```python
from build123d import *

# Parameters (mm, degrees)
F0_R     = 2
F1_DEPTH = 4
F3_DEPTH = 25
F4_R     = 0.99999
F5_DEPTH = 23
F7_START = 24
F6_W     = 30
F6_H     = 37
F7_DEPTH = 6
F9_DEPTH = 25


# Not quite as in the source:
# - a fillet or chamfer is up to 0.001 mm smaller than in the source, because OpenCascade refuses the exact size


with BuildPart() as f1:
    # F0 (on Top) → F1 (new body)
    with BuildSketch(Plane.XY):
        with BuildLine():
            Line((28.5, 21), (-28.5, 21))
            ThreePointArc((-28.5, 21), (-31.3284271247, 19.8284271247), (-32.5, 17))
            Line((-32.5, 17), (-32.5, 8))
            ThreePointArc((-32.5, 8), (-33.6715728753, 5.1715728753), (-36.5, 4))
            ThreePointArc((-36.5, 4), (-40.5, 0), (-36.5, -4))
            ThreePointArc((-36.5, -4), (-33.6715728753, -5.1715728753), (-32.5, -8))
            Line((-32.5, -8), (-32.5, -17))
            ThreePointArc((-32.5, -17), (-31.3284271247, -19.8284271247), (-28.5, -21))
            Line((-28.5, -21), (28.5, -21))
            ThreePointArc((28.5, -21), (31.3284271247, -19.8284271247), (32.5, -17))
            Line((32.5, -17), (32.5, -8))
            ThreePointArc((32.5, -8), (33.6715728753, -5.1715728753), (36.5, -4))
            ThreePointArc((36.5, -4), (40.5, 0), (36.5, 4))
            ThreePointArc((36.5, 4), (33.6715728753, 5.1715728753), (32.5, 8))
            Line((32.5, 8), (32.5, 17))
            ThreePointArc((32.5, 17), (31.3284271247, 19.8284271247), (28.5, 21))
        make_face()
        with Locations((-36.5, 0)):
            Circle(F0_R, mode=Mode.SUBTRACT)
        with BuildLine():
            ThreePointArc((29.5, -16), (28.9142135624, -17.4142135624), (27.5, -18))
            Line((27.5, -18), (-27.5, -18))
            ThreePointArc((-27.5, -18), (-28.9142135624, -17.4142135624), (-29.5, -16))
            Line((-29.5, -16), (-29.5, 16))
            ThreePointArc((-29.5, 16), (-28.9142135624, 17.4142135624), (-27.5, 18))
            Line((-27.5, 18), (27.5, 18))
            ThreePointArc((27.5, 18), (28.9142135624, 17.4142135624), (29.5, 16))
            Line((29.5, 16), (29.5, -16))
        make_face(mode=Mode.SUBTRACT)
        with Locations((36.5, 0)):
            Circle(F0_R, mode=Mode.SUBTRACT)
    extrude(amount=F1_DEPTH)

    # F2 (on Top) → F3 (join)
    with BuildSketch(Plane.XY):
        with BuildLine():
            Line((28, 20), (-28, 20))
            ThreePointArc((-28, 20), (-30.1213203436, 19.1213203436), (-31, 17))
            Line((-31, 17), (-31, -17))
            ThreePointArc((-31, -17), (-30.1213203436, -19.1213203436), (-28, -20))
            Line((-28, -20), (28, -20))
            ThreePointArc((28, -20), (30.1213203436, -19.1213203436), (31, -17))
            Line((31, -17), (31, 17))
            ThreePointArc((31, 17), (30.1213203436, 19.1213203436), (28, 20))
        make_face()
    extrude(amount=F3_DEPTH)

    # F4 (radius 1 in the source; OpenCascade refuses exactly that, so slightly less here)
    f4_edges = [f1.edges().sort_by_distance(p)[0] for p in [
        (0, -20, 4),
        (30.12132, -19.12132, 4),
    ]]
    fillet(f4_edges, radius=F4_R)

    # F0 (on Top) → F5 (cut)
    with BuildSketch(Plane.XY):
        with BuildLine():
            Line((-27.5, -18), (27.5, -18))
            ThreePointArc((27.5, -18), (28.9142135624, -17.4142135624), (29.5, -16))
            Line((29.5, -16), (29.5, 16))
            ThreePointArc((29.5, 16), (28.9142135624, 17.4142135624), (27.5, 18))
            Line((27.5, 18), (-27.5, 18))
            ThreePointArc((-27.5, 18), (-28.9142135624, 17.4142135624), (-29.5, 16))
            Line((-29.5, 16), (-29.5, -16))
            ThreePointArc((-29.5, -16), (-28.9142135624, -17.4142135624), (-27.5, -18))
        make_face()
    extrude(amount=F5_DEPTH, mode=Mode.SUBTRACT)

    # F6 (on Top) → F7 (cut)
    with BuildSketch(Plane.XY.offset(F7_START)):
        Rectangle(F6_W, F6_H)
        Polygon((-4.8068542965, -3.2168254256), (0, 16.6418794543), (5.5426517501, 16.6418794543), (-0.7649944164, 1.0344976326), (8.4538720548, 4.3500550091), (1.9844917115, -10.7721220702), (5.5426517501, -9.3165114522), (-1.4119322877, -17.3223689198), (-1.4119322877, -7.2948294692), (0, -9.8017146811), (0.5527317408, -10.3439353406), (3.8597108796, 0), align=None, mode=Mode.SUBTRACT)
    extrude(amount=F7_DEPTH, mode=Mode.SUBTRACT)

    # F8 (on Front) → F9 (cut)
    with BuildSketch(Plane.XZ):
        with BuildLine():
            Line((3.1964714846, -4.5143875896), (2.9989856559, 3.0780066406))
            ThreePointArc((2.9989856559, 3.0780066406), (-0.0784155915, 5.9989749907), (-2.9989642698, 2.921175459))
            Line((-2.9989642698, 2.921175459), (-2.8035285154, -4.5143875896))
            Line((-2.8035285154, -4.5143875896), (3.1964714846, -4.5143875896))
        make_face()
    extrude(amount=-F9_DEPTH, mode=Mode.SUBTRACT)


solid = f1.part
```
CAD build for the part. Positions are in the model's coordinates, mm. A direction names the side the tool comes from. Round coordinates to 2 decimals unless told otherwise and drop trailing zeros. Order: outer loops, then holes, each group sorted by start corner. A loop starts at its lowest first (then second) coordinate and runs counter-clockwise, first axis right, second up. Notation, with made-up numbers: (80.5, 87.5) - (100.5, 87.5) arc R20 cw to (100.5, 91.5) - close; hole circle Ø1 at (67, 19.25). An arc over 180 degrees is marked (long way). Answer as CSV lines item,"result". Start each with the question number.
1. Pin check, flat tips, straight feed: pin 1 (12.5 mm diameter, centred on x = -5, y = 5, fed in from +Z); pin 2 (11 mm diameter, centred on x = 5, y = 3.5, fed in from -Z); pin 3 (5 mm diameter, centred on y = -14, z = 13, fed in from -X); pin 4 (3 mm diameter, centred on y = 7, z = 4, fed in from +X). Stop position of each tip, or through.
2. Drill centre lines: L1, parallel to Y at x = 36.5, z = 1.25; L2, parallel to X at y = 16, z = 15; L3, parallel to Y at x = -13, z = 18. Where is each one in solid material? Low to high. Write a range as [from, to].
3. Pull direction X, two halves, no side cores. Call faces 1 (the face through (-38.498, 0.088, 1.972)), 2 (the face through (16, 21, 2)), 3 (the face through (0, 0, 23)), 4 (the face through (-31, 0, 15)): +X half, -X half, draft (parallel to the pull), parting line (faces both ways), or undercut.
4. Tool access for faces 5 (the face through (28.93, 17.4, 11.34)), 6 (the face through (30.1, -19.14, 14.86)), 7 (the face through (5.264, -3.105, 24.493)): list every direction of +Z, -Z, +X, -X, +Y, -Y with a clear straight run to the whole face (end or side of a thin tool).
5. Saw through at A-A, the plane z = 8.5. Write the cut outline in (x, y).
6. Saw through at C-C, the plane y = -6. Write the cut outline in (x, z).
Model answer:
1,pin 1,"stops at z = 25"
1,pin 2,"stops at z = 23"
1,pin 3,"stops at x = -31"
1,pin 4,"stops at x = 33.38"
2,L1,"y = [-4, -2], [2, 4]"
2,L2,"x = [-31, -29.5], [29.5, 31]"
2,L3,"y = [-20, -18], [18, 20]"
3,face 1,"undercut"
3,face 2,"draft"
3,face 3,"undercut"
3,face 4,"-X half"
4,face 5,"-Z"
4,face 6,"+Z, +X, -Y"
4,face 7,"+Z"
5,outline,"(-31, -17) arc R3 ccw to (-28, -20) - (28, -20) arc R3 ccw to (31, -17) - (31, 17) arc R3 ccw to (28, 20) - (-28, 20) arc R3 ccw to (-31, 17) - close; hole (-29.5, -16) arc R2 ccw to (-27.5, -18) - (27.5, -18) arc R2 ccw to (29.5, -16) - (29.5, 16) arc R2 ccw to (27.5, 18) - (-27.5, 18) arc R2 ccw to (-29.5, 16) - close"
6,outline,"(-33.04, 0) - (-29.5, 0) - (-29.5, 23) - (29.5, 23) - (29.5, 0) - (33.04, 0) - (33.04, 4) - (32, 4) arc R1 cw to (31, 5) - (31, 25) - (15, 25) - (15, 24) - (4.03, 24) - (4.03, 25) - (1.94, 25) - (1.94, 24) - (-15, 24) - (-15, 25) - (-31, 25) - (-31, 5) arc R1 cw to (-32, 4) - (-33.04, 4) - close"
